Answer from the drawing. Dimensions are ordinates in mm from the lowest x, y and z of the part. A direction names the side the tool comes from. Coordinates: 2 decimals unless noted, no trailing zeros. Write each loop counter-clockwise with the first axis right and the second up, starting at its lowest first coordinate (ties: lowest second). Pieces come first, ordered by that corner, then holes. Notation, with made-up numbers: (-31.5, 7.25) - (-12.5, 7.25) arc R19 ccw to (-12.5, 41.25) - close; hole circle Ø6 at (46, -25). An arc over 180 degrees is marked (long way). Use one line per item in the form item = value. Start each with the question number.
Item 1: A cutting plane is placed at D-D (x = 80). Write down the section's boundary in (y, z), then the cut area to 3 significant figures.
Item 2: Given pin 1 (3 mm diameter, centred on x = 55, z = 2.5, fed in from +Y); pin 2 (10 mm diameter, centred on x = 113, z = 15, fed in from +Y); pin 3 (10 mm diameter, centred on y = 71, z = 8, fed in from -X); pin 4 (4 mm diameter, centred on x = 14.25, z = 10, fed in from -Y), each flat-ended and moving along its own axis, determine where each tip first touches the part or whether it passes through.
Item 3: A cutting plane is placed at A-A (x = 14.25). Write down the section's boundary in (y, z).
Item 4: A cutting plane is placed at B-B (z = 10). Write down the section's boundary in (x, y), then the cut area to 3 significant figures.
Item 5: Consider probe 1 along X at (y, z) = (100.9, 10); probe 2 along X at (y, z) = (68, 11.75); probe 3 along Z at (x, y) = (145.75, 100.7). Determine where each line is inside the solid, lowest interval first.
Item 6: For the marked faces 1, 2, 3 and 4, determine the directions among +Z, -Z, +X, -X, +Y, -Y from which every point of the face is accessible in a straight line to the end or side of a thin tool.
Item 7: A cutting plane is placed at C-C (y = 74.5). Write down the section's boundary in (x, z).
Item 8: Determine the mould class of the marked faces 5, 6 and 7 for opening direction X: released by +X, released by -X, zero draft, split by the parting line, or undercut.
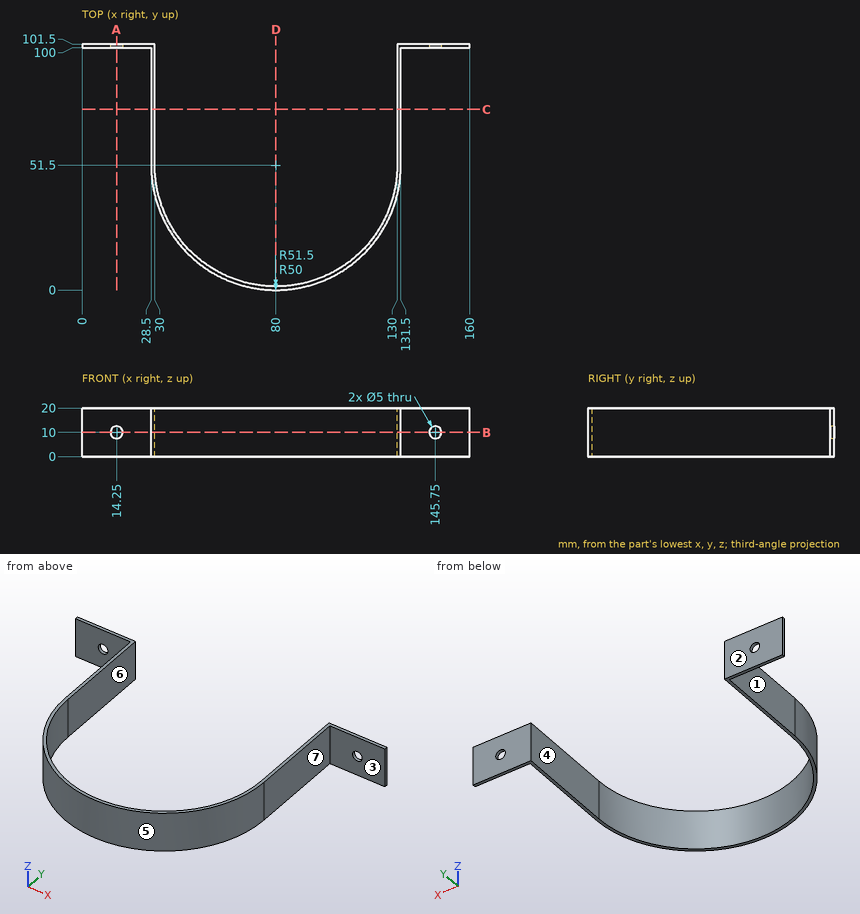
Answer:
q1.outline = (0, 0) - (1.5, 0) - (1.5, 20) - (0, 20) - close
q1.area = 30.0 mm²
q2.pin_1 = 9.1
q2.pin_2 = 19
q2.pin_3 = 28.5
q2.pin_4 = through
q3.outline = (100, 0) - (101.5, 0) - (101.5, 7.5) - (100, 7.5) - close; (100, 12.5) - (101.5, 12.5) - (101.5, 20) - (100, 20) - close
q4.outline = (0, 100) - (11.75, 100) - (11.75, 101.5) - (0, 101.5) - close; (16.75, 100) - (28.5, 100) - (28.5, 51.5) arc R51.5 ccw to (131.5, 51.5) - (131.5, 100) - (143.25, 100) - (143.25, 101.5) - (130, 101.5) - (130, 51.5) arc R50 cw to (30, 51.5) - (30, 101.5) - (16.75, 101.5) - close; (148.25, 100) - (160, 100) - (160, 101.5) - (148.25, 101.5) - close
q4.area = 460 mm²
q5.probe_1 = 0 to 11.75, 16.75 to 30, 130 to 143.25, 148.25 to 160
q5.probe_2 = 28.5 to 30, 130 to 131.5
q5.probe_3 = 0 to 7.5, 12.5 to 20
q6.face_1 = +Z, -Z, -X, -Y
q6.face_2 = +Z, -Z, +X, -X, +Y
q6.face_3 = +Z, -Z, +X, -Y
q6.face_4 = +Z, -Z, +Y
q7.outline = (28.5, 0) - (30, 0) - (30, 20) - (28.5, 20) - close; (130, 0) - (131.5, 0) - (131.5, 20) - (130, 20) - close
q8.face_5 = split by the parting line
q8.face_6 = undercut
q8.face_7 = released by +X
